Geometry check sheet. Reference: the model listing, model coordinates, mm. Face numbers are marked on the shaded views. Give positions to 0.01 mm unless a question says otherwise; leave off trailing zeros. Loops run counter-clockwise (first coordinate to the right, second up) from the corner with the lowest first, then second, coordinate; pieces in that order, holes last. Notation, with made-up numbers: (14, 34.5) - (43, 34.5) arc R20 cw to (43, 41.5) - close; hole circle Ø4 at (84, -21). An arc over 180 degrees is marked (long way). Use a Markdown table: item, result. Add a question column.
1. Cross-section at B-B on y = -10. Enter the section's corners in (x, z) (3 decimals), and give its area (3 significant figures).
2. Draft check along X on the marked faces 1, 2 and 3. Enter one of: pulls with the +X half, pulls with the -X half, needs draft (parallel to the pull), parting line crosses it, or undercut.
3. Cross-section at D-D on y = 21.5. Enter the section's corners in (x, z).
4. Material ranges on L1, parallel to X at y = -10, z = 17.5 (3 decimals); L2, parallel to Y at x = -10.5, z = 7.5, recorded low to high.
5. Depth check by flat-ended pin: P1, Ø4.5, axis at x = 10, y = 10, coming from the +Z side; P2, Ø5, axis at y = 9.5, z = 11, coming from the -X side; P3, Ø3, axis at y = -8.5, z = 16.5, coming from the +X side; P4, Ø5, axis at y = 16, z = 17, coming from the -X side. Enter the tip coordinate at first touch or a pass-through.
6. Cross-section at A-A on z = 3.75. Enter the section's corners in (x, y).
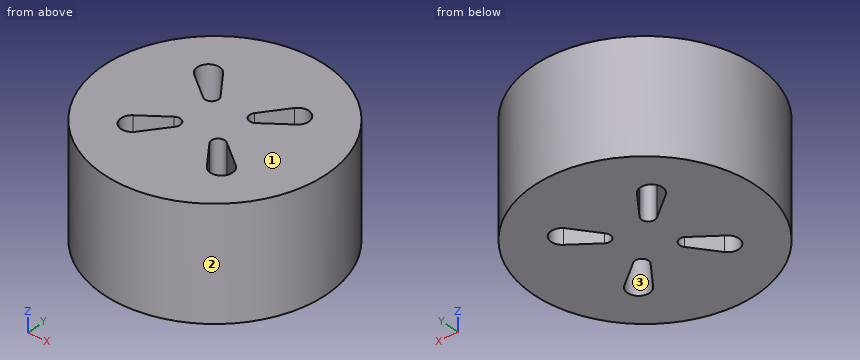
from build123d import *

# Parameters (mm, degrees)
F0_R     = 25
F1_DEPTH = 25


with BuildPart() as f1:
    # F0 (on Top) → F1 (new body)
    with BuildSketch(Plane.XY):
        Circle(F0_R)
        with BuildLine():
            Line((-11.5, -8), (-5.9, -3.8))
            ThreePointArc((-5.9, -3.8), (-3.93934, -3.93934), (-3.8, -5.9))
            Line((-3.8, -5.9), (-8, -11.5))
            ThreePointArc((-8, -11.5), (-11.767767, -11.767767), (-11.5, -8))
        make_face(mode=Mode.SUBTRACT)
        with BuildLine():
            ThreePointArc((11.5, -8), (11.767767, -11.767767), (8, -11.5))
            Line((8, -11.5), (3.8, -5.9))
            ThreePointArc((3.8, -5.9), (3.93934, -3.93934), (5.9, -3.8))
            Line((5.9, -3.8), (11.5, -8))
        make_face(mode=Mode.SUBTRACT)
        with BuildLine():
            ThreePointArc((-11.5, 8), (-11.767767, 11.767767), (-8, 11.5))
            Line((-8, 11.5), (-3.8, 5.9))
            ThreePointArc((-3.8, 5.9), (-3.93934, 3.93934), (-5.9, 3.8))
            Line((-5.9, 3.8), (-11.5, 8))
        make_face(mode=Mode.SUBTRACT)
        with BuildLine():
            Line((3.8, 5.9), (8, 11.5))
            ThreePointArc((8, 11.5), (11.767767, 11.767767), (11.5, 8))
            Line((11.5, 8), (5.9, 3.8))
            ThreePointArc((5.9, 3.8), (3.93934, 3.93934), (3.8, 5.9))
        make_face(mode=Mode.SUBTRACT)
    extrude(amount=F1_DEPTH)


solid = f1.part
Values found:
| question | item | result |
|---|---|---|
| 1 | outline | (-22.913, 0) - (-12.5, 0) - (-12.5, 25) - (-22.913, 25) - close; (-6.875, 0) - (6.875, 0) - (6.875, 25) - (-6.875, 25) - close; (12.5, 0) - (22.913, 0) - (22.913, 25) - (12.5, 25) - close |
| 1 | area | 864 mm2 |
| 2 | face 1 | needs draft |
| 2 | face 2 | parting line crosses it |
| 2 | face 3 | undercut |
| 3 | outline | (-12.76, 0) - (12.76, 0) - (12.76, 25) - (-12.76, 25) - close |
| 4 | L1 | x = -22.913 to -12.5, -6.875 to 6.875, 12.5 to 22.913 |
| 4 | L2 | y = -22.69 to -12.45, -7.25 to 7.25, 12.45 to 22.69 |
| 5 | P1 | passes through |
| 5 | P2 | stops at x = -24 |
| 5 | P3 | stops at x = 24 |
| 5 | P4 | stops at x = -21.04 |
| 6 | outline | circle Ø50 at (0, 0); hole (-11.5, -8) arc R2.5 ccw (long way) to (-8, -11.5) - (-3.8, -5.9) arc R1.5 ccw to (-5.9, -3.8) - close; hole (-11.5, 8) - (-5.9, 3.8) arc R1.5 ccw to (-3.8, 5.9) - (-8, 11.5) arc R2.5 ccw (long way) to start; hole (3.8, -5.9) - (8, -11.5) arc R2.5 ccw (long way) to (11.5, -8) - (5.9, -3.8) arc R1.5 ccw to start; hole (3.8, 5.9) arc R1.5 ccw to (5.9, 3.8) - (11.5, 8) arc R2.5 ccw (long way) to (8, 11.5) - close |
